Check sheet for the modelled part. Datum: model origin and axes. Units: mm. A direction names the side the tool comes from. Give positions to 0.01 mm unless a question says otherwise; leave off trailing zeros. Write each loop counter-clockwise with the first axis right and the second up, starting at its lowest first coordinate (ties: lowest second). Pieces come first, ordered by that corner, then holes. Notation, with made-up numbers: (14, 2.5) - (40, 2.5) arc R36 cw to (40, 41.5) - close; hole circle Ø5 at (84, -7.75). An arc over 180 degrees is marked (long way). Return JSON: item names as keys, results as strings. Group by question number.
```python
from build123d import *

# Parameters (mm, degrees)
SKETCH1_R               = 16.5
BOSS_EXTRUDE1_DEPTH     = 10
SKETCH2_R               = 3.05
CUT_EXTRUDE1_DEPTH      = 1.25
SKETCH4_W               = 4.95
SKETCH4_H               = 5.75
CUT_EXTRUDE2_DEPTH      = 25.921125577
CUT_EXTRUDE2_DEPTH_BACK = 25.921125577
SKETCH5_R               = 2


with BuildPart() as part:
    # Sketch1 → Boss-Extrude1 (new body)
    with BuildSketch(Plane(origin=(0, 0, 0), x_dir=(1, 0, 0), z_dir=(0, 1, 0))):
        with Locations(Location((0, 0, 0), (0, 0, 270))):
            Circle(SKETCH1_R)
    extrude(amount=BOSS_EXTRUDE1_DEPTH)

    # Sketch2 → Cut-Extrude1 (cut)
    with BuildSketch(Plane(origin=(0, 10, 0), x_dir=(1, 0, 0), z_dir=(0, 1, 0))):
        with Locations(Location((0, 0, 0), (0, 0, 270))):
            Circle(SKETCH2_R)
    extrude(amount=-CUT_EXTRUDE1_DEPTH, mode=Mode.SUBTRACT)

    # Sketch4 → Revolve1 (revolve)
    with BuildSketch(Plane.XY, mode=Mode.PRIVATE) as revolve1_sk:
        with Locations((8.975, 12.875)):
            Rectangle(SKETCH4_W, SKETCH4_H)
    revolve(revolve1_sk.sketch.rotate(Axis((0, -0.517946451, 0), (0, 1, 0)), 90), axis=Axis((0, -0.517946451, 0), (0, 1, 0)))

    # Sketch5 → Cut-Extrude2 (cut, two sides: drawn at the far end of the back side and taken through both)
    with BuildSketch(Plane(origin=(0, 8.75, 0), x_dir=(1, 0, 0), z_dir=(0, 1, 0)).offset(-CUT_EXTRUDE2_DEPTH_BACK)):
        with Locations(Location((0, 0, 0), (0, 0, 270))):
            Circle(SKETCH5_R)
    extrude(amount=CUT_EXTRUDE2_DEPTH + CUT_EXTRUDE2_DEPTH_BACK, mode=Mode.SUBTRACT)


solid = part.part
```
Item 1: Access from +Z, -Z, +X, -X, +Y, -Y to the whole of each face (thin tool, end or side, straight path). Record for faces 1 (the face through (-16.108, 4.93, -3.577)), 2 (the face through (2, 10, 3)).
Item 2: Depth check by flat-ended pin: pin 1 (3 mm diameter, centred on x = 2, y = 2.5, fed in from -Z); pin 2 (1.8 mm diameter, centred on x = 0, z = -1.5, fed in from +Y); pin 3 (6 mm diameter, centred on y = 4, z = 4.5, fed in from -X). Enter the tip coordinate at first touch or a pass-through.
Item 3: Section check A-A on z = 0. Record the cut outline in (x, y).
Item 4: Section check C-C on y = 4.5. Record the cut outline in (x, z).
Item 5: Section check B-B on x = 0. Record the cut outline in (y, z).
Item 6: Material ranges on line 1 along X through (y, z) = (6.5, 0); line 2 along X through (y, z) = (11.7, 0); line 3 along Y through (x, z) = (7.5, -12), recorded low to high. Write a range as from..to.
Item 7: Mould release check, pull along Z, two halves, no side actions. Record for faces 3 (the face through (11.18, 12.92, 2.48)), 4 (the face through (-2, 4, 0)), 5 (the face through (-3, 0, 0)): +Z half, -Z half, draft (parallel to the pull), parting line (faces both ways), or undercut.
Item 8: Section check D-D on z = -4. Record the cut outline in (x, y), plus the area to 3 significant figures.
Reply:
{
 "1": {"face 1": "+Y, -Y", "face 2": "+Y"},
 "2": {"pin 1": "z = -16.49", "pin 2": "y = 8.75", "pin 3": "x = -16.43"},
 "3": {"outline": "(-16.5, 0) - (-2, 0) - (-2, 8.75) - (-3.05, 8.75) - (-3.05, 10) - (-6.5, 10) - (-6.5, 15.75) - (-11.45, 15.75) - (-11.45, 10) - (-16.5, 10) - close; (2, 0) - (16.5, 0) - (16.5, 10) - (11.45, 10) - (11.45, 15.75) - (6.5, 15.75) - (6.5, 10) - (3.05, 10) - (3.05, 8.75) - (2, 8.75) - close"},
 "4": {"outline": "circle Ø33 at (0, 0); hole circle Ø4 at (0, 0)"},
 "5": {"outline": "(0, -16.5) - (10, -16.5) - (10, -11.45) - (15.75, -11.45) - (15.75, -6.5) - (10, -6.5) - (10, -3.05) - (8.75, -3.05) - (8.75, -2) - (0, -2) - close; (0, 2) - (8.75, 2) - (8.75, 3.05) - (10, 3.05) - (10, 6.5) - (15.75, 6.5) - (15.75, 11.45) - (10, 11.45) - (10, 16.5) - (0, 16.5) - close"},
 "6": {"line 1": "-16.5..-2, 2..16.5", "line 2": "-11.45..-6.5, 6.5..11.45", "line 3": "0..10"},
 "7": {"face 3": "parting line", "face 4": "undercut", "face 5": "draft"},
 "8": {"outline": "(-16.01, 0) - (16.01, 0) - (16.01, 10) - (10.73, 10) - (10.73, 15.75) - (5.12, 15.75) - (5.12, 10) - (-5.12, 10) - (-5.12, 15.75) - (-10.73, 15.75) - (-10.73, 10) - (-16.01, 10) - close", "area": "385 mm²"}
}
